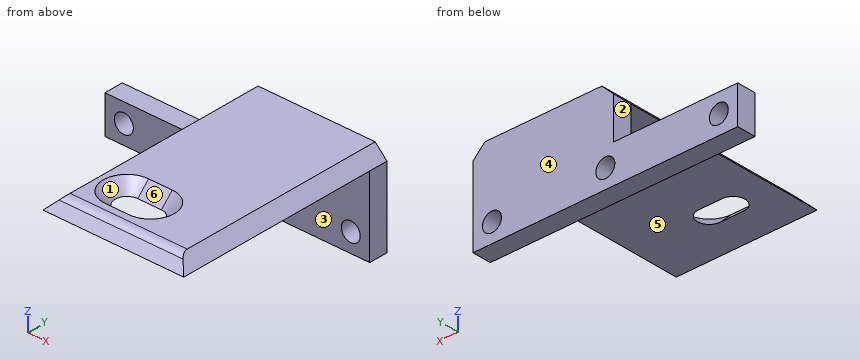
Autodesk Inventor part; units mm, degrees
ref_plane "YZ Plane" through (0, 0, 0) normal (1, 0, 0) x (0, 1, 0)
ref_plane "XZ Plane" through (0, 0, 0) normal (0, 1, 0) x (-1, 0, 0)
ref_plane "XY Plane" through (0, 0, 0) normal (0, 0, 1) x (1, 0, 0)
sketch "Sketch1" plane through (0, 0, 0) normal (0, 1, 0) x (-1, 0, 0)
  line L0 (0, 0) -> (-19.17, 0)
  circle A0 centre (0, 0) radius 1.6
  circle A1 centre (-19.17, 0) radius 1.6
  line L1 (-19.17, 0) -> (-22.37, 0)
  line L2 (0, 0) -> (3.2, 0)
  line L3 (-22.37, 0) -> (-22.37, 3.2)
  line L4 (3.2, 0) -> (3.2, -3.2)
  line L5 (3.2, -3.2) -> (-22.37, -3.2)
  line L6 (-22.37, -3.2) -> (-22.37, 3.2)
  line L7 (-22.37, 3.2) -> (3.2, 3.2)
  line L8 (3.2, 3.2) -> (3.2, -3.2)
  line L9 (3.2, 3.2) -> (3.2, 10.2)
  line L10 (3.2, 10.2) -> (3.2, 12.2)
  line L11 (3.2, 12.2) -> (-22.37, 12.2)
  line L12 (-22.37, 12.2) -> (-22.37, 10.2)
  line L13 (-22.37, 10.2) -> (3.2, 10.2)
  line L14 (-22.37, 3.2) -> (-22.37, 10.2)
  line L15 (-9.585, 12.2) -> (1.415, 12.2)
  line L16 (-9.585, 12.2) -> (-15.985, 12.2)
  line L17 (-15.985, 12.2) -> (-15.985, 10.2)
  line L18 (1.415, 12.2) -> (1.415, 10.2)
  line L19 (0, 0) -> (0, -3.2)
  circle A2 centre (19.17, 0) radius 1.6
  line L20 (22.37, 0) -> (22.37, 3.2)
  line L21 (-3.2, 0) -> (-3.2, -3.2)
  line L22 (-3.2, -3.2) -> (22.37, -3.2)
  line L23 (22.37, -3.2) -> (22.37, 3.2)
  line L24 (22.37, 3.2) -> (-3.2, 3.2)
  line L25 (-3.2, 3.2) -> (-3.2, -3.2)
  line L26 (3.2, 10.2) -> (8.2, 10.2)
  line L27 (8.2, 10.2) -> (8.2, 3.2)
  line L28 (8.2, 10.2) -> (8.2, 12.2)
  line L29 (8.2, 12.2) -> (3.2, 12.2)
  line L30 (1.415, 10.2) -> (1.415, 3.2)
  line L31 (-15.985, 10.2) -> (-15.985, 3.2)
  point P0 (3.2, 3.2)
  point P1 (3.2, 3.2)
  point P2 (1.415, 3.2)
  dimension "d0" = 19.17
  dimension "d1" = 3.2
  dimension "d2" = 3.2
  dimension "d3" = 3.2
  dimension "d4" = 3.2
  dimension "d5" = 3.2
  dimension "d6" = 3.2
  dimension "d7" = 7
  dimension "d8" = 2
  dimension "d21" = 11
  dimension "d22" = 6.4
  dimension "d30" = 5
extrude "Extrusion1" add sketch "Sketch1" along normal blind 6.4 contours L17 L11 L18 L13 | L13 L12 L11 L17
extrude "Extrusion2" add sketch "Sketch1" along normal blind 3.2 from surface at 6.4 contours L21 L5 L6 L1 A1 L0 | L25 L7 L8 L2 A0 L0 | L0 A0 L19 L5 L21 | L0 A1 L1 L3 L7 L25 | L7 L31 L13 L30 | L2 L4 L5 L19 A0 | L7 L14 L13 L31 | L8 L24 L20 L23 L22 L4 | L17 L11 L18 L13 | L13 L12 L11 L17
extrude "Extrusion3" add sketch "Sketch1" against normal blind 28 contours L17 L11 L18 L13 | L13 L12 L11 L17
sketch "Sketch2" plane through (-3.2, 9.6, 12.2) normal (0, 0, 1) x (1, 0, 0)
  line L0 (0, 0) -> (0, -9.6)
  line L1 (0, -9.6) -> (0, -29.6)
  line L2 (-3.2, -29.6) -> (21.33, -29.6)
  line L3 (9.065, -30.1) -> (5.865, -30.1)
  line L4 (9.065, -29.6) -> (12.265, -29.6)
  line L5 (0, -3.2) -> (0, 0)
  line L6 (0, 0) -> (0, -9.6)
  arc A0 (8.665, -27.6) -> (8.665, -31.6) centre (8.665, -29.6) ccw
  line L7 (8.665, -27.6) -> (12.665, -27.6)
  line L8 (12.665, -31.6) -> (8.665, -31.6)
  arc A1 (12.665, -31.6) -> (12.665, -27.6) centre (12.665, -29.6) ccw
  point P0 (3.2, -9.6)
  point P1 (0, -30.1)
  dimension "d16" = 20
  dimension "d18" = 3.2
  dimension "d23" = 9.6
extrude "Extrusion4" cut sketch "Sketch2" against normal through all
chamfer "Chamfer2" distance 2 angle 45 7 edges at (7.465, -18, 12.2) (11.465, -20, 12.2) (7.465, -22, 12.2) (3.465, -20, 12.2) (22.37, -9.2, 12.2) (10.4775, -28, 12.2) (-1.415, -9.2, 12.2)
fillet "Fillet2" radius 2 1 edges at (10.4775, -26.0005, 12.2)
properties part number "enclosure mounter"
The model under review builds one solid part; all positions refer to its coordinate system, in mm. Face numbers are marked on the shaded views. A direction names the side the tool comes from. Coordinates: 2 decimals unless noted, no trailing zeros. Loops run counter-clockwise (first coordinate to the right, second up) from the corner with the lowest first, then second, coordinate; pieces in that order, holes last. Notation, with made-up numbers: (-11.75, 75.25) -> (8.25, 75.25) arc R19 ccw to (8.25, 104.25) -> close; hole circle Ø4 at (84.25, 9.25). An arc over 180 degrees is marked (long way). Use a Markdown table: item, result. Add a question column.
1. To check wall thickness, follow line 1 (Z direction, x = -19, y = 8); line 2 (Z direction, x = 0, y = 7.1); line 3 (Y direction, x = 3.5, z = 3.5). State the ranges of each line that lie inside material, in increasing order.
2. Draft analysis for pull direction Y (two halves, no side actions). For the marked faces 4, 5 and 6, state which applies: pulls with the +Y half, pulls with the -Y half, needs draft (parallel to the pull), parting line crosses it, or undercut.
3. Add section B-B on z = 0. Write out the cut boundary in (x, y), plus the area to 3 significant figures.
4. Add section A-A on x = -19.17. Write out the cut boundary in (y, z).
5. Machinability: for the marked faces 1, 2 and 3, which of the approach directions +Z, -Z, +X, -X, +Y, -Y give a long, thin tool a straight path to every point of the face, cutting with its end or side? Answer none if there is none.
6. Clearance check with flat-ended pins moving along their axes: pin 1 Ø3 at (x, z) = (11.5, 9) entering from -Y; pin 2 Ø4 at (x, z) = (-1.5, 9.5) entering from +Y; pin 3 Ø1 at (x, y) = (18, -5) entering from -Z; pin 4 Ø5.5 at (y, z) = (-11, 7.5) entering from -X (3 decimals). State where each tip first meets the part, or that it passes through.
Returned:
| question | item | result |
|---|---|---|
| 1 | line 1 | z = -3.2 to -1.59, 1.59 to 3.2 |
| 1 | line 2 | z = -3.2 to -1.6, 1.6 to 11.62 |
| 1 | line 3 | y = 6.4 to 9.6 |
| 2 | face 4 | pulls with the +Y half |
| 2 | face 5 | needs draft |
| 2 | face 6 | undercut |
| 3 | outline | (-22.37, 6.4) -> (-20.77, 6.4) -> (-20.77, 9.6) -> (-22.37, 9.6) -> close; (-17.57, 6.4) -> (-1.6, 6.4) -> (-1.6, 9.6) -> (-17.57, 9.6) -> close; (1.6, 6.4) -> (17.57, 6.4) -> (17.57, 9.6) -> (1.6, 9.6) -> close; (20.77, 6.4) -> (22.37, 6.4) -> (22.37, 9.6) -> (20.77, 9.6) -> close |
| 3 | area | 112 mm² |
| 4 | outline | (6.4, -3.2) -> (9.6, -3.2) -> (9.6, -1.6) -> (6.4, -1.6) -> close; (6.4, 1.6) -> (9.6, 1.6) -> (9.6, 3.2) -> (6.4, 3.2) -> close |
| 5 | face 1 | +Z |
| 5 | face 2 | +Z, -X, +Y, -Y |
| 5 | face 3 | -Z, +X, -X, -Y |
| 6 | pin 1 | stops at y = -28 |
| 6 | pin 2 | stops at y = 9.6 |
| 6 | pin 3 | stops at z = 10.2 |
| 6 | pin 4 | stops at x = -1.415 |
